from build123d import *

# Parameters (mm, degrees)
SKETCH1_R           = 67.25
SKETCH1_R_2         = 59.5
BOSS_EXTRUDE1_DEPTH = 20
SKETCH4_R           = 3.175
CUT_EXTRUDE2_DEPTH  = 200
SKETCH5_R           = 4.826
CUT_EXTRUDE3_DEPTH  = 4
SKETCH6_R           = 6.35
CUT_EXTRUDE4_DEPTH  = 1


with BuildPart() as part:
    # Sketch1 → Boss-Extrude1 (new body)
    with BuildSketch(Plane(origin=(0, 0, 0), x_dir=(1, 0, 0), z_dir=(0, 1, 0))):
        with Locations(Location((0, 0, 0), (0, 0, 270))):
            Circle(SKETCH1_R)
        with Locations(Location((0, 0, 0), (0, 0, 270))):
            Circle(SKETCH1_R_2, mode=Mode.SUBTRACT)
    extrude(amount=BOSS_EXTRUDE1_DEPTH)

    # Sketch4 → Cut-Extrude2 (cut)
    with BuildSketch(Plane(origin=(67.25, 0, 0), x_dir=(0, 0, -1), z_dir=(1, 0, 0))):
        with Locations((0, 10)):
            Circle(SKETCH4_R)
    extrude(amount=-CUT_EXTRUDE2_DEPTH, mode=Mode.SUBTRACT)

    # Sketch5 → Cut-Extrude3 (cut)
    with BuildSketch(Plane(origin=(67.25, 0, 0), x_dir=(0, 0, -1), z_dir=(1, 0, 0))):
        with Locations((0, 10)):
            Circle(SKETCH5_R)
    cut_extrude3 = extrude(amount=-CUT_EXTRUDE3_DEPTH, mode=Mode.SUBTRACT)

    # Mirror1: Cut-Extrude3 across plane
    add(cut_extrude3.mirror(Plane(origin=(0, 0, 0), x_dir=(0, 0, 1), z_dir=(1, 0, 0))), mode=Mode.SUBTRACT)

    # Sketch6 → Cut-Extrude4 (cut, symmetric)
    with BuildSketch(Plane(origin=(59.45, 0, 0), x_dir=(0, 0, -1), z_dir=(1, 0, 0))):
        with Locations(Location((0, 10, 0), (0, 0, 180))):
            Circle(SKETCH6_R)
    cut_extrude4 = extrude(amount=CUT_EXTRUDE4_DEPTH, both=True, mode=Mode.SUBTRACT)

    # Mirror2: Cut-Extrude4 across plane
    add(cut_extrude4.mirror(Plane(origin=(0, 0, 0), x_dir=(0, 0, 1), z_dir=(1, 0, 0))), mode=Mode.SUBTRACT)


solid = part.part
Here's how the part is built. I have some questions about the finished solid (model axes, mm). A direction names the side the tool comes from. Coordinates: 2 decimals unless noted, no trailing zeros. Write each loop counter-clockwise with the first axis right and the second up, starting at its lowest first coordinate (ties: lowest second). Pieces come first, ordered by that corner, then holes.
1) If we section it at D-D (y = 10): List the corners of the cut face in (x, z) for me (3 decimals).
Filled in:
outline: (-67.077, -4.826) arc R67.25 ccw to (67.077, -4.826) - (63.25, -4.826) - (63.25, -3.175) - (60.45, -3.175) - (60.45, -6.35) - (59.16, -6.35) arc R59.5 cw to (-59.16, -6.35) - (-60.45, -6.35) - (-60.45, -3.175) - (-63.25, -3.175) - (-63.25, -4.826) - close; (-67.077, 4.826) - (-63.25, 4.826) - (-63.25, 3.175) - (-60.45, 3.175) - (-60.45, 6.35) - (-59.16, 6.35) arc R59.5 cw to (59.16, 6.35) - (60.45, 6.35) - (60.45, 3.175) - (63.25, 3.175) - (63.25, 4.826) - (67.077, 4.826) arc R67.25 ccw to start
2) If we section it at A-A (z = 0): Count the separate pieces of the cut face and the enclosed holes in it, plus the area to 3 significant figures.
Filled in:
separate pieces: 4
enclosed holes: 0
area: 173 mm2
3) Thinking about a two-plate mould opening in Y: for faces 6 (the face through (-59.5, 20, 4.7)), 7 (the face through (-63.25, 11.14, -3.15)), 8 (the face through (-59.5, 0, 4.7)), which applies, +Y half, -Y half, draft (parallel to the pull), parting line (faces both ways), or undercut?
Filled in:
face 6: +Y half
face 7: undercut
face 8: -Y half
4) If we section it at B-B (x = 0): List the corners of the cut face in (y, z) for me.
Filled in:
outline: (0, -67.25) - (20, -67.25) - (20, -59.5) - (0, -59.5) - close; (0, 59.5) - (20, 59.5) - (20, 67.25) - (0, 67.25) - close
5) If I drill on line 1 (X direction, y = 16.5, z = -1.5); line 2 (Y direction, x = -62, z = 0) (3 decimals); line 3 (X direction, y = 14.25, z = 0), over which ranges is the centre line in solid material (lowest first)?
Filled in:
line 1: x = -67.23 to -59.48, 59.48 to 67.23
line 2: y = 0 to 6.825, 13.175 to 20
line 3: x = -63.25 to -60.45, 60.45 to 63.25
6) If we section it at C-C (z = -42): List the corners of the cut face in (x, y) for me.
Filled in:
outline: (-52.52, 0) - (-42.15, 0) - (-42.15, 20) - (-52.52, 20) - close; (42.15, 0) - (52.52, 0) - (52.52, 20) - (42.15, 20) - close
7) Which directions (+Z, -Z, +X, -X, +Y, -Y) give clear straight access to the entire face, cutting with the end or side of a thin tool? Please do faces 1 (the face through (63.25, 11.14, -3.15)), 2 (the face through (-61.83, 6.9, 0.69)), 3 (the face through (-59.662, 9.86, 31.032)), 4 (the face through (-65.278, 14.785, 0.628)), 5 (the face through (59.957, 12.432, 5.866)).
Filled in:
face 1: +X
face 2: +X, -X
face 3: +Y, -Y
face 4: -X
face 5: none
8) I'm going to push flat-ended pins straight in: pin 1 (4 mm diameter, centred on y = 12, z = -1.5, fed in from -X); pin 2 (4 mm diameter, centred on x = 31.5, y = 13, fed in from -Z); pin 3 (6 mm diameter, centred on x = 33, y = 11.5, fed in from +Z); pin 4 (5.5 mm diameter, centred on y = 10, z = 0, fed in from -X). Where does each tip first touch, or does it pass through?
Filled in:
pin 1: stops at x = -63.25
pin 2: stops at z = -60.43
pin 3: stops at z = 60.19
pin 4: passes through
